```python
from build123d import *

# Parameters (mm, degrees)
F0_R     = 38.1
F1_DEPTH = 50.8
F2_R     = 6.35
F3_DEPTH = 70.612
F4_R     = 5.08


with BuildPart() as f1:
    # F0 (on Top) → F1 (new body)
    with BuildSketch(Plane.XY):
        Circle(F0_R)
    extrude(amount=F1_DEPTH)

    # F2 (on face) → F3 (cut)
    with BuildSketch(Plane.XY.offset(50.8)):
        with Locations((0, 7.62)):
            Circle(F2_R)
        with Locations((0, -7.62)):
            Circle(F2_R)
    extrude(amount=-F3_DEPTH, mode=Mode.SUBTRACT)

    # F4
    f4_edges = [f1.edges().sort_by_distance(p)[0] for p in [
        (-38.1, 0, 50.8),
    ]]
    fillet(f4_edges, radius=F4_R)


solid = f1.part
```
CAD build for the part. Positions are in the model's coordinates, mm. Round coordinates to 2 decimals unless told otherwise and drop trailing zeros. Order: outer loops, then holes, each group sorted by start corner. A loop starts at its lowest first (then second) coordinate and runs counter-clockwise, first axis right, second up. Notation, with made-up numbers: (31.25, 1) - (85.25, 1) arc R19 cw to (85.25, 9) - close; hole circle Ø10 at (53.5, 18.25). An arc over 180 degrees is marked (long way). Use CSV: the item, a comma, the result in double quotes. Start each with the question number.
1) Saw through at A-A (x = 0). List the corners of the cut face in (y, z).
2) Pin check, flat tips, straight feed: pin 1 Ø1.5 at (y, z) = (4.5, 32.5) entering from +X (3 decimals); pin 2 Ø1 at (y, z) = (25, 25.5) entering from -X; pin 3 Ø10 at (x, z) = (-14, 23.5) entering from -Y. Stop position of each tip, or through.
3) Wall check: L1, parallel to Y at x = 0, z = 35.5; L2, parallel to X at y = 5, z = 25.5; L3, parallel to X at y = 11, z = 37. Give the ranges that are in metal, low to high. Write a range as [from, to].
4) Two-plate mould, pull along Y, no slides. Class faces 1 (the flat face through (0, 0, 50.8)), 2 (the cylindrical face through (-30.235, -23.183, 22.54)), 3 (the cylindrical face through (-1.38, -13.82, 25.76)): pulls with the +Y half, pulls with the -Y half, needs draft (parallel to the pull), parting line crosses it, or undercut.
5) Saw through at B-B (z = 6). List the corners of the cut face in (x, y), and give its area (3 significant figures).
Values follow:
1,outline,"(-38.1, 0) - (-13.97, 0) - (-13.97, 50.8) - (-33.02, 50.8) arc R5.08 ccw to (-38.1, 45.72) - close; (-1.27, 0) - (1.27, 0) - (1.27, 50.8) - (-1.27, 50.8) - close; (13.97, 0) - (38.1, 0) - (38.1, 45.72) arc R5.08 ccw to (33.02, 50.8) - (13.97, 50.8) - close"
2,pin 1,"stops at x = 37.915"
2,pin 2,"stops at x = -29.18"
2,pin 3,"stops at y = -37.02"
3,L1,"y = [-38.1, -13.97], [-1.27, 1.27], [13.97, 38.1]"
3,L2,"x = [-37.77, -5.78], [5.78, 37.77]"
3,L3,"x = [-36.48, -5.38], [5.38, 36.48]"
4,face 1,"needs draft"
4,face 2,"parting line crosses it"
4,face 3,"undercut"
5,outline,"circle Ø76.2 at (0, 0); hole circle Ø12.7 at (0, -7.62); hole circle Ø12.7 at (0, 7.62)"
5,area,"4,310 mm2"
